```python
from build123d import *

# Parameters (mm, degrees)
F0_W     = 9
F0_H     = 80
F1_DEPTH = 4
F0_W_2   = 4
F2_DEPTH = 18
F3_START = 14
F3_DEPTH = 4


with BuildPart() as f1:
    # F0 (on Top) → F1 (new body)
    with BuildSketch(Plane.XY):
        with Locations((-6.5, 0)):
            Rectangle(F0_W, F0_H)
        with BuildLine():
            ThreePointArc((-9.25, 36), (-7, 38.25), (-4.75, 36))
            Line((-4.75, 36), (-4.75, -36))
            ThreePointArc((-4.75, -36), (-7, -38.25), (-9.25, -36))
            Line((-9.25, -36), (-9.25, 36))
        make_face(mode=Mode.SUBTRACT)
    extrude(amount=F1_DEPTH)

    # F0 (on Top) → F2 (join)
    with BuildSketch(Plane.XY):
        Rectangle(F0_W_2, F0_H)
    extrude(amount=F2_DEPTH)

    # F0 (on Top) → F3 (join)
    with BuildSketch(Plane.XY.offset(F3_START)):
        with Locations((6.5, 0)):
            Rectangle(F0_W, F0_H)
        with BuildLine():
            ThreePointArc((4.75, 36), (7, 38.25), (9.25, 36))
            Line((9.25, 36), (9.25, -36))
            ThreePointArc((9.25, -36), (7, -38.25), (4.75, -36))
            Line((4.75, -36), (4.75, 36))
        make_face(mode=Mode.SUBTRACT)
    extrude(amount=F3_DEPTH)


solid = f1.part
```
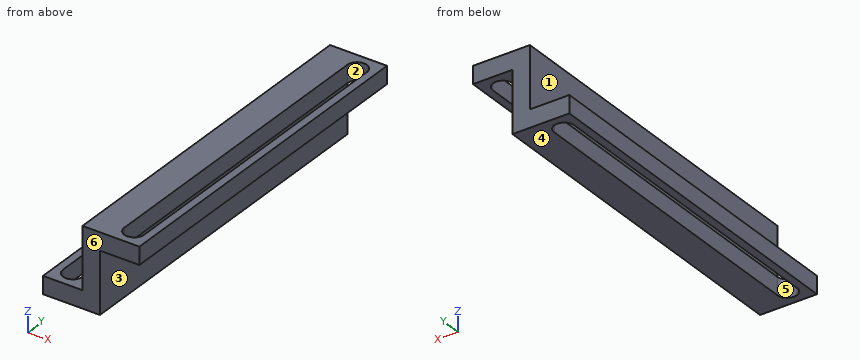
CAD build for the part. Positions are in the model's coordinates, mm. Face numbers are marked on the shaded views. A direction names the side the tool comes from. Coordinates: 2 decimals unless noted, no trailing zeros. Write each loop counter-clockwise with the first axis right and the second up, starting at its lowest first coordinate (ties: lowest second). Pieces come first, ordered by that corner, then holes.
(1) Flat gauge pins, fed straight in: pin 1 (2.5 mm diameter, centred on x = -5.5, y = -3.5, fed in from +Z); pin 2 (2 mm diameter, centred on y = -1, z = 17, fed in from -X); pin 3 (4 mm diameter, centred on y = -12, z = 4, fed in from +X). Where does each tip first touch, or does it go through?
(2) Cut at A-A, the plane y = -4. List the corners of the cut face in (x, z).
(3) 3-axis set-ups, long thin cutter, end or side, ignore diameter. For the marked faces 5 and 6: which of +Z, -Z, +X, -X, +Y, -Y reach the whole face in a straight line?
(4) Drill centre lines: probe 1 along X at (y, z) = (-30, 17); probe 2 along X at (y, z) = (-10.5, 3); probe 3 along X at (y, z) = (-34, 8). Where is each one in solid material? Low to high.
(5) Cut at B-B, the plane x = -7. List the corners of the cut face in (y, z), and give its area (3 significant figures).
(6) Cut at C-C, the plane z = 3.25. List the corners of the cut face in (x, y), and give its area (3 significant figures).
(7) Cut at D-D, the plane x = 3. List the corners of the cut face in (y, z), and give its area (3 significant figures).
(8) Two-plate mould, pull along X, no slides. Class the marked faces 1, 2, 3 and 4: +X half, -X half, draft (parallel to the pull), parting line (faces both ways), or undercut.
Geometry says:
1. pin 1: stops at z = 4
1. pin 2: stops at x = -2
1. pin 3: stops at x = 2
2. outline: (-11, 0) - (-9.25, 0) - (-9.25, 4) - (-11, 4) - close; (-4.75, 0) - (2, 0) - (2, 14) - (4.75, 14) - (4.75, 18) - (-2, 18) - (-2, 4) - (-4.75, 4) - close; (9.25, 14) - (11, 14) - (11, 18) - (9.25, 18) - close
3. face 5: +Z, -Z
3. face 6: +Z, -Z, +X, -X, -Y
4. probe 1: x = -2 to 4.75, 9.25 to 11
4. probe 2: x = -11 to -9.25, -4.75 to 2
4. probe 3: x = -2 to 2
5. outline: (-40, 0) - (-38.25, 0) - (-38.25, 4) - (-40, 4) - close; (38.25, 0) - (40, 0) - (40, 4) - (38.25, 4) - close
5. area: 14.0 mm2
6. outline: (-11, -40) - (2, -40) - (2, 40) - (-11, 40) - close; hole (-9.25, -36) arc R2.25 ccw to (-4.75, -36) - (-4.75, 36) arc R2.25 ccw to (-9.25, 36) - close
6. area: 700 mm2
7. outline: (-40, 14) - (40, 14) - (40, 18) - (-40, 18) - close
7. area: 320 mm2
8. face 1: -X half
8. face 2: undercut
8. face 3: +X half
8. face 4: draft
